Verification items for the finished model (mm, model axes). Round coordinates to 2 decimals unless told otherwise and drop trailing zeros. Order: outer loops, then holes, each group sorted by start corner. A loop starts at its lowest first (then second) coordinate and runs counter-clockwise, first axis right, second up. Notation, with made-up numbers: (-38, 35.5) -> (-22, 35.5) arc R26 cw to (-22, 59.5) -> close; hole circle Ø7 at (-7, 2). An arc over 180 degrees is marked (long way). Put each result on its own line as item: value.
```python
from build123d import *

# Parameters (mm, degrees)
CROQUIS1_R                 = 1.5
SALIENTE_EXTRUIR1_DEPTH    = 2
CORTAR_EXTRUIR1_DEPTH      = 96.880459427
CORTAR_EXTRUIR1_DEPTH_BACK = 2


with BuildPart() as part:
    # Croquis1 → Saliente-Extruir1 (new body)
    with BuildSketch(Plane.XY):
        with BuildLine():
            Line((-17, 88.75), (17, 88.75))
            ThreePointArc((17, 88.75), (19.121320344, 87.871320344), (20, 85.75))
            Line((20, 85.75), (20, -90.75))
            ThreePointArc((20, -90.75), (19.121320344, -92.871320344), (17, -93.75))
            Line((17, -93.75), (-17, -93.75))
            ThreePointArc((-17, -93.75), (-19.121320344, -92.871320344), (-20, -90.75))
            Line((-20, -90.75), (-20, 85.75))
            ThreePointArc((-20, 85.75), (-19.121320344, 87.871320344), (-17, 88.75))
        make_face()
        with Locations((-16, 84.25)):
            Circle(CROQUIS1_R, mode=Mode.SUBTRACT)
        with Locations((16, 84.25)):
            Circle(CROQUIS1_R, mode=Mode.SUBTRACT)
        with Locations((-16, 41.25)):
            Circle(CROQUIS1_R, mode=Mode.SUBTRACT)
        with Locations((16, 41.25)):
            Circle(CROQUIS1_R, mode=Mode.SUBTRACT)
        with Locations((-16, -11.75)):
            Circle(CROQUIS1_R, mode=Mode.SUBTRACT)
        with Locations((16, -11.75)):
            Circle(CROQUIS1_R, mode=Mode.SUBTRACT)
        with Locations((-16, -89.25)):
            Circle(CROQUIS1_R, mode=Mode.SUBTRACT)
        with Locations((16, -89.25)):
            Circle(CROQUIS1_R, mode=Mode.SUBTRACT)
    extrude(amount=SALIENTE_EXTRUIR1_DEPTH)

    # Croquis2 → Cortar-Extruir1 (cut, two sides: drawn at the far end of the back side and taken through both)
    with BuildSketch(Plane.XY.offset(2).offset(-CORTAR_EXTRUIR1_DEPTH_BACK)):
        with BuildLine():
            ThreePointArc((-12.400415076, 88.75), (-11.253262204, 88.388304089), (-10.521029835, 87.434040287))
            Line((-10.521029835, 87.434040287), (-8.931178525, 83.065959713))
            ThreePointArc((-8.931178525, 83.065959713), (-8.198946156, 82.111695911), (-7.051793284, 81.75))
            Line((-7.051793284, 81.75), (7.051793284, 81.75))
            ThreePointArc((7.051793284, 81.75), (8.198946156, 82.111695911), (8.931178525, 83.065959713))
            Line((8.931178525, 83.065959713), (10.521029835, 87.434040287))
            ThreePointArc((10.521029835, 87.434040287), (11.253262204, 88.388304089), (12.400415076, 88.75))
            Line((12.400415076, 88.75), (-12.400415076, 88.75))
        make_face()
    extrude(amount=CORTAR_EXTRUIR1_DEPTH + CORTAR_EXTRUIR1_DEPTH_BACK, mode=Mode.SUBTRACT)


solid = part.part
```
Item 1: Sectioned sample at B-B, the plane z = 0.4. Give the number of separate pieces and of enclosed holes in the cut face, then the cut area to 3 significant figures.
Geometry check:
separate pieces: 1
enclosed holes: 8
area: 7,100 mm2
Item 2: Material ranges on line 1 along Y through (x, z) = (-16, 1.55); line 2 along X through (y, z) = (-89.25, 1.4); line 3 along X through (y, z) = (84.25, 1.45), recorded low to high.
Geometry check:
line 1: -93.75 to -90.75, -87.75 to -13.25, -10.25 to 39.75, 42.75 to 82.75, 85.75 to 88.75
line 2: -20 to -17.5, -14.5 to 14.5, 17.5 to 20
line 3: -20 to -17.5, -14.5 to -9.36, 9.36 to 14.5, 17.5 to 20
Item 3: Release check for a two-part mould opening along X. For faces 1 (the face through (19.1, 87.89, 0.99)), 2 (the face through (-19.14, 87.85, 0.99)), 3 (the face through (14.5, -11.7, 1)) record: pulls with the +X half, pulls with the -X half, needs draft (parallel to the pull), parting line crosses it, or undercut.
Geometry check:
face 1: pulls with the +X half
face 2: pulls with the -X half
face 3: undercut
Item 4: Sectioned sample at A-A, the plane y = 41.25. Record the boundary of the cut face in (x, z), then the cut area to 3 significant figures.
Geometry check:
outline: (-20, 0) -> (-17.5, 0) -> (-17.5, 2) -> (-20, 2) -> close; (-14.5, 0) -> (14.5, 0) -> (14.5, 2) -> (-14.5, 2) -> close; (17.5, 0) -> (20, 0) -> (20, 2) -> (17.5, 2) -> close
area: 68.0 mm2
Item 5: Depth check by flat-ended pin: pin 1 Ø1.8 at (x, y) = (-16, 84.25) entering from -Z. Enter the tip coordinate at first touch or a pass-through.
Geometry check:
pin 1: through
